Geometry: final body of the model. Coordinates: model frame, mm. Give positions to 0.01 mm unless a question says otherwise; leave off trailing zeros. Loops run counter-clockwise (first coordinate to the right, second up) from the corner with the lowest first, then second, coordinate; pieces in that order, holes last. Notation, with made-up numbers: (49, 74) - (106, 74) arc R26 ccw to (106, 111) - close; hole circle Ø6 at (25, 69.5). An arc over 180 degrees is marked (long way). Answer in a Markdown table with one row per item.
from build123d import *

# Parameters (mm, degrees)
SKETCH_1_W      = 50
SKETCH_1_H      = 20
SKETCH_1_R      = 2
EXTRUDE_1_DEPTH = 4
FILLET_1_R      = 10


with BuildPart() as part:
    # 草图1 → 凸台-拉伸1 (new body)
    with BuildSketch(Plane.XY):
        with Locations((25, -10)):
            Rectangle(SKETCH_1_W, SKETCH_1_H)
        with Locations((7, -10)):
            Circle(SKETCH_1_R, mode=Mode.SUBTRACT)
        with Locations((19, -10)):
            Circle(SKETCH_1_R, mode=Mode.SUBTRACT)
        with Locations((31, -10)):
            Circle(SKETCH_1_R, mode=Mode.SUBTRACT)
        with Locations((43, -10)):
            Circle(SKETCH_1_R, mode=Mode.SUBTRACT)
    extrude(amount=EXTRUDE_1_DEPTH)

    # 圆角1
    fillet_1_edges = [part.edges().sort_by_distance(p)[0] for p in [
        (50, 0, 2),
        (50, -20, 2),
        (0, -20, 2),
        (0, 0, 2),
    ]]
    fillet(fillet_1_edges, radius=FILLET_1_R - 0.0001)  # a hair under: the kernel refuses the full size


solid = part.part
Q1. Cut plane A-A (x = 19). Output: boundary loops of the cut face in (y, z).
Check values:
| item | result |
|---|---|
| outline | (-20, 0) - (-12, 0) - (-12, 4) - (-20, 4) - close; (-8, 0) - (0, 0) - (0, 4) - (-8, 4) - close |
Q2. Cut plane C-C (x = 7). Output: boundary loops of the cut face in (y, z).
Check values:
| item | result |
|---|---|
| outline | (-19.54, 0) - (-12, 0) - (-12, 4) - (-19.54, 4) - close; (-8, 0) - (-0.46, 0) - (-0.46, 4) - (-8, 4) - close |
Q3. Cut plane D-D (y = -2.75). Output: boundary loops of the cut face in (x, z), and give its area (3 significant figures).
Check values:
| item | result |
|---|---|
| outline | (3.11, 0) - (46.89, 0) - (46.89, 4) - (3.11, 4) - close |
| area | 175 mm² |
Q4. First-contact query: pin 1 (3 mm diameter, centred on x = 7, y = -10, fed in from -Z); pin 2 (2 mm diameter, centred on y = -15, z = 1, fed in from +X). Flat tips, straight axial feed; report the tip coordinate or a pass-through.
Check values:
| item | result |
|---|---|
| pin 1 | through |
| pin 2 | x = 49.17 |
Q5. Cut plane B-B (z = 2.55). Give the number of separate pieces and of enclosed holes in the cut face, and give its area (3 significant figures).
Check values:
| item | result |
|---|---|
| separate pieces | 1 |
| enclosed holes | 4 |
| area | 864 mm² |
Q6. Material intervals for line 1 along Y through (x, z) = (19, 1.7); line 2 along Y through (x, z) = (30.5, 2.4); line 3 along X through (y, z) = (-3, 1.7), sorted ascending.
Check values:
| item | result |
|---|---|
| line 1 | -20 to -12, -8 to 0 |
| line 2 | -20 to -11.94, -8.06 to 0 |
| line 3 | 2.86 to 47.14 |
